Geometry check sheet. Reference: the model listing, model coordinates, mm. Face numbers are marked on the shaded views. A direction names the side the tool comes from. Coordinates: 2 decimals unless noted, no trailing zeros. Write each loop counter-clockwise with the first axis right and the second up, starting at its lowest first coordinate (ties: lowest second). Pieces come first, ordered by that corner, then holes. Notation, with made-up numbers: (84.25, 43) -> (105.25, 43) arc R32 cw to (105.25, 72) -> close; hole circle Ø6 at (12, 78.25). An arc over 180 degrees is marked (long way). One line per question, with ' | ' between items.
from build123d import *

# Parameters (mm, degrees)
EXTRUDE_1_DEPTH     = 10
SKETCH_3_R          = 1.6
CUT_EXTRUDE_1_DEPTH = 5
SKETCH_2_R          = 1.6
CUT_EXTRUDE_2_DEPTH = 5
FILLET_1_R          = 0.5


with BuildPart() as part:
    # Sketch 1 → 凸台-拉伸1 (new body)
    with BuildSketch(Plane.XY):
        Polygon((0, 15), (0, 0), (15, 0), (15, 3), (3, 3), (3, 15), align=None)
    extrude(amount=EXTRUDE_1_DEPTH)

    # 草图3 → 切除-拉伸1 (cut)
    with BuildSketch(Plane.XZ):
        with Locations(Location((10, 5, 0), (0, 0, 270))):
            Circle(SKETCH_3_R)
    extrude(amount=-CUT_EXTRUDE_1_DEPTH, mode=Mode.SUBTRACT)

    # Sketch 2 → 切除-拉伸2 (cut)
    with BuildSketch(Plane.ZY):
        with Locations(Location((5, 10, 0), (0, 0, 270))):
            Circle(SKETCH_2_R)
    extrude(amount=-CUT_EXTRUDE_2_DEPTH, mode=Mode.SUBTRACT)

    # 圆角1
    fillet_1_edges = [part.edges().sort_by_distance(p)[0] for p in [
        (3, 15, 5),
        (3, 3, 5),
        (15, 3, 5),
        (15, 0, 5),
        (0, 0, 5),
        (0, 15, 5),
        (7.5, 0, 10),
        (15, 1.5, 10),
        (9, 3, 10),
        (3, 9, 10),
        (1.5, 15, 10),
        (3, 9, 0),
        (9, 3, 0),
        (15, 1.5, 0),
        (7.5, 0, 0),
        (0, 7.5, 0),
        (1.5, 15, 0),
        (0, 7.5, 10),
    ]]
    fillet(fillet_1_edges, radius=FILLET_1_R)


solid = part.part
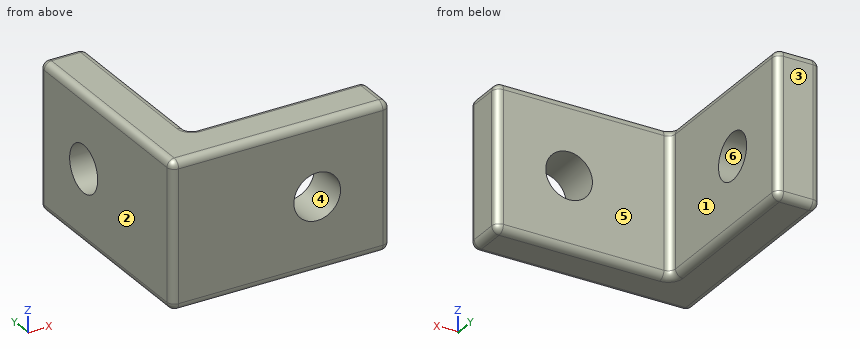
1. Go/stop test with flat-tipped pins: P1, Ø2.5, axis at y = 7.5, z = 5.5, coming from the +X side; P2, Ø3, axis at x = 10, z = 5, coming from the -Y side. Record where each tip stops, or that it passes through.
Worked answers:
P1: x = 3 | P2: through
2. Mould release check, pull along X, two halves, no side actions. Record for the marked faces 1, 2, 3 and 4: released by +X, released by -X, zero draft, split by the parting line, or undercut.
Worked answers:
face 1: released by +X | face 2: released by -X | face 3: zero draft | face 4: undercut
3. Cross-section at B-B on z = 5. Record the boundary of the cut face in (x, y).
Worked answers:
outline: (0, 0.5) arc R0.5 ccw to (0.5, 0) -> (8.4, 0) -> (8.4, 3) -> (3.5, 3) arc R0.5 cw to (3, 3.5) -> (3, 8.4) -> (0, 8.4) -> close; (0, 11.6) -> (3, 11.6) -> (3, 14.5) arc R0.5 ccw to (2.5, 15) -> (0.5, 15) arc R0.5 ccw to (0, 14.5) -> close; (11.6, 0) -> (14.5, 0) arc R0.5 ccw to (15, 0.5) -> (15, 2.5) arc R0.5 ccw to (14.5, 3) -> (11.6, 3) -> close
4. Cross-section at C-C on y = 1.5. Record the boundary of the cut face in (x, z), and give its area (3 significant figures).
Worked answers:
outline: (0, 0.5) arc R0.5 ccw to (0.5, 0) -> (14.5, 0) arc R0.5 ccw to (15, 0.5) -> (15, 9.5) arc R0.5 ccw to (14.5, 10) -> (0.5, 10) arc R0.5 ccw to (0, 9.5) -> close; hole circle Ø3.2 at (10, 5) | area: 142 mm²
5. Tool access check on the marked faces 5 and 6. Record the directions out of +Z, -Z, +X, -X, +Y, -Y that give a thin tool (end or side, any length) a straight path to the whole face; none if there is none.
Worked answers:
face 5: +Z, -Z, +X, +Y | face 6: +X, -X
6. Cross-section at A-A on y = 10. Record the boundary of the cut face in (x, z).
Worked answers:
outline: (0, 0.5) arc R0.5 ccw to (0.5, 0) -> (2.5, 0) arc R0.5 ccw to (3, 0.5) -> (3, 3.4) -> (0, 3.4) -> close; (0, 6.6) -> (3, 6.6) -> (3, 9.5) arc R0.5 ccw to (2.5, 10) -> (0.5, 10) arc R0.5 ccw to (0, 9.5) -> close
7. Material ranges on line 1 (X direction, y = 0.7, z = 5); line 2 (Z direction, x = 1.2, y = 10); line 3 (X direction, y = 4.75, z = 8.75), recorded low to high. Write a range as from..to.
Worked answers:
line 1: 0..8.4, 11.6..15 | line 2: 0..3.4, 6.6..10 | line 3: 0..3
